Geometry: final body of the model. Coordinates: model frame, mm. Give positions to 0.01 mm unless a question says otherwise; leave off trailing zeros. Loops run counter-clockwise (first coordinate to the right, second up) from the corner with the lowest first, then second, coordinate; pieces in that order, holes last.
1. First-contact query: P1, Ø1.5, axis at y = -3, z = 1, coming from the -X side; P2, Ø1, axis at y = -15.5, z = 0.5, coming from the +X side; P3, Ø0.9, axis at x = 34, z = 1, coming from the -Y side. Flat tips, straight axial feed; report the tip coordinate or a pass-through.
2. Material intervals for line 1 along X through (y, z) = (3, 2.8); line 2 along X through (y, z) = (23.5, 1.1); line 3 along Y through (x, z) = (40.5, 2), sorted ascending.
3. Section C-C, the plane z = 1.8. State how many separate pieces and enclosed holes the cut face has, then the cut area to 3 significant figures.
4. Section A-A, the plane y = 13. Output: boundary loops of the cut face in (x, z), then the cut area to 3 significant figures.
5. Section B-B, the plane x = 23. Output: boundary loops of the cut face in (y, z), then the cut area to 3 significant figures.
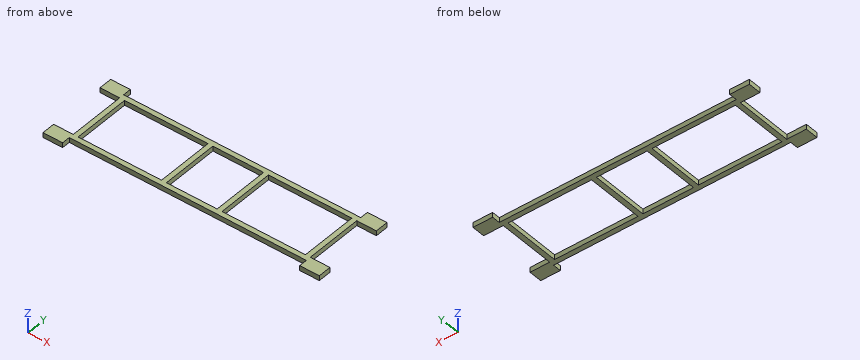
from build123d import *

# Parameters (mm, degrees)
F0_W     = 169
F0_H     = 51
F1_DEPTH = 3
F2_W     = 51
F2_H     = 35
F2_W_2   = 12
F2_W_3   = 72.5
F2_H_2   = 5
F2_W_4   = 15.5
F3_DEPTH = 3


# Not quite as in the source:
# - a pattern or mirror of a feature is missing from the dataset's text; its kind, count and spacing are read off the source's solid


with BuildPart() as f1:
    # F0 (on Top) → F1 (new body)
    with BuildSketch(Plane.XY):
        Rectangle(F0_W, F0_H)
    extrude(amount=F1_DEPTH)

    # F2 (on face) → F3 (cut, through all)
    with BuildSketch(Plane.XY.offset(3)):
        with Locations((-44, 0)):
            Rectangle(F2_W, F2_H)
        with Locations((-78.5, 0)):
            Rectangle(F2_W_2, F2_H)
        with Locations((-36.25, 23)):
            Rectangle(F2_W_3, F2_H_2)
        with Locations((-36.25, -23)):
            Rectangle(F2_W_3, F2_H_2)
        with Locations((-7.75, 0)):
            Rectangle(F2_W_4, F2_H)
    f3 = extrude(amount=-F3_DEPTH, mode=Mode.SUBTRACT)

    # F3_copies: F3 across plane
    add(f3.mirror(Plane(origin=(0, 0, 0), x_dir=(0, 0, 1), z_dir=(1, 0, 0))), mode=Mode.SUBTRACT)


solid = f1.part
Answers below:
1. P1: stops at x = -72.5
1. P2: stops at x = 72.5
1. P3: stops at y = -20.5
2. line 1: x = -72.5 to -69.5, -18.5 to -15.5, 15.5 to 18.5, 69.5 to 72.5
2. line 2: x = -84.5 to -72.5, 72.5 to 84.5
2. line 3: y = -20.5 to -17.5, 17.5 to 20.5
3. separate pieces: 1
3. enclosed holes: 3
3. area: 1,670 mm2
4. outline: (-72.5, 0) - (-69.5, 0) - (-69.5, 3) - (-72.5, 3) - close; (-18.5, 0) - (-15.5, 0) - (-15.5, 3) - (-18.5, 3) - close; (15.5, 0) - (18.5, 0) - (18.5, 3) - (15.5, 3) - close; (69.5, 0) - (72.5, 0) - (72.5, 3) - (69.5, 3) - close
4. area: 36.0 mm2
5. outline: (-20.5, 0) - (-17.5, 0) - (-17.5, 3) - (-20.5, 3) - close; (17.5, 0) - (20.5, 0) - (20.5, 3) - (17.5, 3) - close
5. area: 18.0 mm2
